Part model, mm, in its own coordinate system. Face numbers are marked on the shaded views. Coordinates: 2 decimals unless noted, no trailing zeros. Write each loop counter-clockwise with the first axis right and the second up, starting at its lowest first coordinate (ties: lowest second). Pieces come first, ordered by that corner, then holes. Notation, with made-up numbers: (60.25, 13.25) -> (81.25, 13.25) arc R23 cw to (81.25, 29.25) -> close; hole circle Ø2 at (64, -16.5). An arc over 180 degrees is marked (long way). Write item = value, one per line. Start each with the question number.
Q1. Probe line 1 (X direction, y = 38.5, z = -10); line 2 (X direction, y = 35.5, z = -14); line 3 (Z direction, x = 180, y = 27.5). List the from-to ranges inside material, lowest first.
Q2. Band-saw the part on C-C, the plane z = -18.5. List the corners of the cut face in (x, y).
Q3. Band-saw the part on B-B, the plane z = -10. List the corners of the cut face in (x, y), plus the area to 3 significant figures.
Q4. Band-saw the part on D-D, the plane x = 128. List the corners of the cut face in (y, z).
Q5. Band-saw the part on A-A, the plane x = 180. List the corners of the cut face in (y, z).
Q6. Pin check, flat tips, straight feed: P1, Ø3, axis at x = 178, z = -9, coming from the -Y side; P2, Ø6, axis at x = 224.5, y = 28, coming from the +Z side; P3, Ø4, axis at x = 219.5, z = -13.5, coming from the -Y side. Stop position of each tip, or through.
Q7. Pull direction Z, two halves, no side cores. Call the marked faces 1, 2 and 3: released by +Z, released by -Z, zero draft, split by the parting line, or undercut.
from build123d import *

# Parameters (mm, degrees)
SKETCH_1_W          = 120
SKETCH_1_H          = 20
EXTRUDE_1_DEPTH     = 50
SKETCH_2_W          = 6
SKETCH_2_H          = 20
EXTRUDE_2_DEPTH     = 20
CUT_EXTRUDE_1_DEPTH = 114
SKETCH_4_R          = 2.6
SKETCH_4_W          = 20
SKETCH_4_H          = 20
CUT_EXTRUDE_2_DEPTH = 114
SKETCH_5_R          = 5
CUT_EXTRUDE_3_DEPTH = 3
CUT_EXTRUDE_4_DEPTH = 300
SKETCH_8_R          = 5
CUT_EXTRUDE_5_DEPTH = 300
SKETCH_9_R          = 5
SKETCH_9_R_2        = 2.6
EXTRUDE_3_DEPTH     = 3
SKETCH_11_W         = 120
SKETCH_11_H         = 20
CUT_EXTRUDE_6_DEPTH = 100
CUT_EXTRUDE_7_DEPTH = 10


# Read off the part's stored shape, not the designer's step: the mirror step
with BuildPart() as part:
    # Sketch 1 → Extrude 1 (new body)
    with BuildSketch(Plane(origin=(0, 0, 0), x_dir=(1, 0, 0), z_dir=(0, 1, 0))):
        with Locations((60, 10)):
            Rectangle(SKETCH_1_W, SKETCH_1_H)
    extrude(amount=EXTRUDE_1_DEPTH)

    # Sketch 2 → Extrude 2 (add)
    with BuildSketch(Plane.XY):
        with Locations((3, -10)):
            Rectangle(SKETCH_2_W, SKETCH_2_H)
    extrude(amount=-EXTRUDE_2_DEPTH)

    # Sketch 3 → Cut-Extrude 1 (cut)
    with BuildSketch(Plane(origin=(120, 0, 0), x_dir=(0, 0, -1), z_dir=(1, 0, 0))):
        Polygon((0, 50), (20, 0), (0, 0), align=None)
    extrude(amount=-CUT_EXTRUDE_1_DEPTH, mode=Mode.SUBTRACT)

    # Sketch 4 → Cut-Extrude 2 (cut)
    with BuildSketch(Plane(origin=(6, 0, 0), x_dir=(0, 0, -1), z_dir=(1, 0, 0))):
        with Locations(Location((10, 10, 0), (0, 0, 90))):
            Circle(SKETCH_4_R)
        with Locations((10, -10)):
            Rectangle(SKETCH_4_W, SKETCH_4_H)
    extrude(amount=-CUT_EXTRUDE_2_DEPTH, mode=Mode.SUBTRACT)

    # Sketch 5 → Cut-Extrude 3 (cut)
    with BuildSketch(Plane(origin=(6, 0, 0), x_dir=(0, 0, -1), z_dir=(1, 0, 0))):
        with Locations(Location((10, 10, 0), (0, 0, 90))):
            Circle(SKETCH_5_R)
    extrude(amount=-CUT_EXTRUDE_3_DEPTH, mode=Mode.SUBTRACT)

    # Sketch 6 → Cut-Extrude 4 (cut)
    with BuildSketch(Plane(origin=(0, 50, 0), x_dir=(1, 0, 0), z_dir=(0, 1, 0))):
        with BuildLine():
            ThreePointArc((62.6, 10), (61.838477631, 11.838477631), (60, 12.6))
            Line((60, 12.6), (60, 7.4))
            ThreePointArc((60, 7.4), (61.838477631, 8.161522369), (62.6, 10))
        make_face()
        with BuildLine():
            Line((60, 7.4), (60, 12.6))
            ThreePointArc((60, 12.6), (57.4, 10), (60, 7.4))
        make_face()
    extrude(amount=-CUT_EXTRUDE_4_DEPTH, mode=Mode.SUBTRACT)

    # Sketch 8 → Cut-Extrude 5 (cut)
    with BuildSketch(Plane(origin=(0, 50, 0), x_dir=(1, 0, 0), z_dir=(0, 1, 0))):
        with Locations(Location((60, 10, 0), (0, 0, 270))):
            Circle(SKETCH_8_R)
    extrude(amount=-CUT_EXTRUDE_5_DEPTH, mode=Mode.SUBTRACT)

    # Sketch 9 → Extrude 3 (add)
    with BuildSketch(Plane(origin=(0, 50, 0), x_dir=(1, 0, 0), z_dir=(0, 1, 0))):
        with Locations(Location((60, 10, 0), (0, 0, 270))):
            Circle(SKETCH_9_R)
        with Locations(Location((60, 10, 0), (0, 0, 270))):
            Circle(SKETCH_9_R_2, mode=Mode.SUBTRACT)
    extrude(amount=-EXTRUDE_3_DEPTH)

    # Mirror 2: part across plane


with BuildPart() as part_1:
    add(part.part)
    add(part.part.mirror(Plane(origin=(120, 50, 0), x_dir=(0, 0, 1), z_dir=(-1, 0, 0))))

    # Sketch 11 → Cut-Extrude 6 (cut)
    with BuildSketch(Plane(origin=(0, 50, 0), x_dir=(1, 0, 0), z_dir=(0, 1, 0))):
        with Locations((60, 10)):
            Rectangle(SKETCH_11_W, SKETCH_11_H)
    extrude(amount=-CUT_EXTRUDE_6_DEPTH, mode=Mode.SUBTRACT)

    # Sketch 12 → Cut-Extrude 7 (cut)
    with BuildSketch(Plane.ZY.offset(-234)):
        Polygon((-20, 0), (0, 0), (0, 50), align=None)
    extrude(amount=-CUT_EXTRUDE_7_DEPTH, mode=Mode.SUBTRACT)


solid = part_1.part
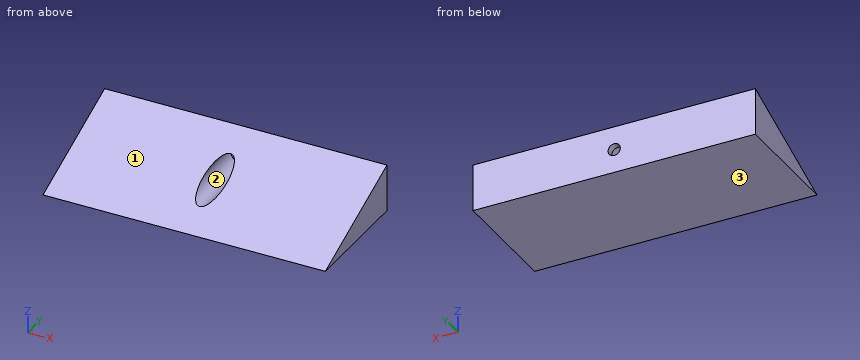
Ans:
q1.line_1 = 120 to 175, 185 to 240
q1.line_2 = 120 to 177, 183 to 240
q1.line_3 = -20 to -15
q2.outline = (120, 3.75) -> (240, 3.75) -> (240, 50) -> (120, 50) -> close
q3.outline = (120, 25) -> (175, 25) -> (175, 47) -> (177.4, 47) -> (177.4, 50) -> (120, 50) -> close; (182.6, 47) -> (185, 47) -> (185, 25) -> (240, 25) -> (240, 50) -> (182.6, 50) -> close
q3.area = 2,760 mm2
q4.outline = (0, -20) -> (50, -20) -> (50, 0) -> close
q5.outline = (0, -20) -> (50, -20) -> (50, -12.6) -> (47, -12.6) -> (47, -15) -> (12.5, -15) -> close; (37.5, -5) -> (47, -5) -> (47, -7.4) -> (50, -7.4) -> (50, 0) -> close
q6.P1 = 47
q6.P2 = -7.6
q6.P3 = 11.25
q7.face_1 = released by +Z
q7.face_2 = undercut
q7.face_3 = released by -Z
